from build123d import *

# Parameters (mm, degrees)
ESQUISSE1_W                                        = 15
ESQUISSE1_H                                        = 16
EXTRUSION1_DEPTH                                   = 10
CHANFREIN1_SIZE                                    = 1
CHAMBRAGE_POUR_VIS_T_TE_HEXAGONALE_M31_D           = 3.4
CHAMBRAGE_POUR_VIS_T_TE_HEXAGONALE_M31_CBORE_D     = 6.5
CHAMBRAGE_POUR_VIS_T_TE_HEXAGONALE_M31_CBORE_DEPTH = 3
ESQUISSE2_W                                        = 5.5288305
ESQUISSE2_H                                        = 4.608549318
ENL_VEMENT_DE_MATI_RE_R_VOLUTION1_ANGLE            = 39
CHANFREIN2_SIZE                                    = 1


with BuildPart() as part:
    # Esquisse1 → Extrusion1 (new body)
    with BuildSketch(Plane.XY):
        with Locations((7.5, 0)):
            Rectangle(ESQUISSE1_W, ESQUISSE1_H)
    extrude(amount=EXTRUSION1_DEPTH)

    # Chanfrein1
    chanfrein1_edges = [part.edges().sort_by_distance(p)[0] for p in [
        (7.5, 8, 10),
        (7.5, -8, 10),
    ]]
    chamfer(chanfrein1_edges, length=CHANFREIN1_SIZE)

    # Chambrage pour vis à tête hexagonale M31 (through all)
    with Locations(Plane(origin=(10.126877496, 0, 10), x_dir=(1, 0, 0), z_dir=(0, 0, 1))):
        with Locations((0, 0)):
            CounterBoreHole(CHAMBRAGE_POUR_VIS_T_TE_HEXAGONALE_M31_D / 2, CHAMBRAGE_POUR_VIS_T_TE_HEXAGONALE_M31_CBORE_D / 2, CHAMBRAGE_POUR_VIS_T_TE_HEXAGONALE_M31_CBORE_DEPTH)

    # Esquisse2 → Enlèvement de matière-Révolution1 (revolve, symmetric, cut)
    with BuildSketch(Plane(origin=(0, 0, 0), x_dir=(1, 0, 0), z_dir=(0, 1, 0))) as enl_vement_de_mati_re_r_volution1_sk:
        with Locations((1.521286307, -6.093228571)):
            Rectangle(ESQUISSE2_W, ESQUISSE2_H)
    revolve(axis=Axis((6.580325396, 0, -22), (1, 0, 0)), revolution_arc=ENL_VEMENT_DE_MATI_RE_R_VOLUTION1_ANGLE / 2, mode=Mode.SUBTRACT)
    revolve(enl_vement_de_mati_re_r_volution1_sk.sketch, axis=Axis((6.580325396, 0, -22), (-1, 0, 0)), revolution_arc=ENL_VEMENT_DE_MATI_RE_R_VOLUTION1_ANGLE / 2, mode=Mode.SUBTRACT)

    # Chanfrein2
    chanfrein2_edges = [part.edges().sort_by_distance(p)[0] for p in [
        (15, 0, 10),
    ]]
    chamfer(chanfrein2_edges, length=CHANFREIN2_SIZE)


solid = part.part
Design review of the part built by this model. Coordinates are the model's own, in mm. A direction names the side the tool comes from. Give positions to 0.01 mm unless a question says otherwise; leave off trailing zeros. Loops run counter-clockwise (first coordinate to the right, second up) from the corner with the lowest first, then second, coordinate; pieces in that order, holes last. Notation, with made-up numbers: (43.5, 15) - (102.5, 15) arc R23 cw to (102.5, 46) - close; hole circle Ø3 at (34, 11.5). An arc over 180 degrees is marked (long way). Write item = value, one per line.
1) Draft analysis for pull direction X (two halves, no side actions). For faces 1 (the face through (0, 0, 2)), 2 (the face through (14.5, -0.1, 9.5)), 3 (the face through (12, -1, 7)), 4 (the face through (7, 0, 0)), state which applies: +X half, -X half, draft (parallel to the pull), parting line (faces both ways), or undercut.
Result sheet:
face_1 = -X half
face_2 = +X half
face_3 = undercut
face_4 = draft
2) Take a section at D-D on y = -4.5. State the section outline as (x, z) points.
Result sheet:
outline = (0, 0) - (15, 0) - (15, 9) - (14, 10) - (0, 10) - (0, 8.06) - (4.29, 8.06) - (4.29, 3.39) - (0, 3.39) - close
3) Clearance check with a flat-ended pin moving along its axis: pin 1 Ø2 at (x, y) = (11.5, 0) entering from +Z. State where the tip first meets the part, or that it passes through.
Result sheet:
pin_1 = 7
4) Tool access review of faces 5 (the face through (2.17, -0.11, 3.79)), 6 (the face through (7.55, -1.98, 8.52)), 7 (the face through (15, 0, 4)): name each direction out of +Z, -Z, +X, -X, +Y, -Y from which nothing blocks a thin tool from reaching the whole face with its end or side.
Result sheet:
face_5 = -X
face_6 = +Z
face_7 = +Z, -Z, +X, +Y, -Y
5) To check wall thickness, follow line 1 (Y direction, x = 11.25, z = 3); line 2 (Z direction, x = 4, y = -1.5); line 3 (Z direction, x = 7, y = 0.25). State the ranges of each line that lie inside material, in increasing order.
Result sheet:
line_1 = -8 to -1.28, 1.28 to 8
line_2 = 0 to 3.75, 8.36 to 10
line_3 = 0 to 7
6) Take a section at A-A on y = 0. State the section outline as (x, z) points.
Result sheet:
outline = (0, 0) - (8.43, 0) - (8.43, 7) - (6.88, 7) - (6.88, 10) - (0, 10) - (0, 8.4) - (4.29, 8.4) - (4.29, 3.79) - (0, 3.79) - close; (11.83, 0) - (15, 0) - (15, 9) - (14, 10) - (13.38, 10) - (13.38, 7) - (11.83, 7) - close
7) Take a section at C-C on x = 7.5. State the section outline as (y, z) points.
Result sheet:
outline = (-8, 0) - (8, 0) - (8, 9) - (7, 10) - (1.91, 10) - (1.91, 7) - (-1.91, 7) - (-1.91, 10) - (-7, 10) - (-8, 9) - close
8) Take a section at B-B on z = 1.5. State the section outline as (x, y) points, and give its area (3 significant figures).
Result sheet:
outline = (0, -8) - (15, -8) - (15, 8) - (0, 8) - close; hole circle Ø3.4 at (10.13, 0)
area = 231 mm2
